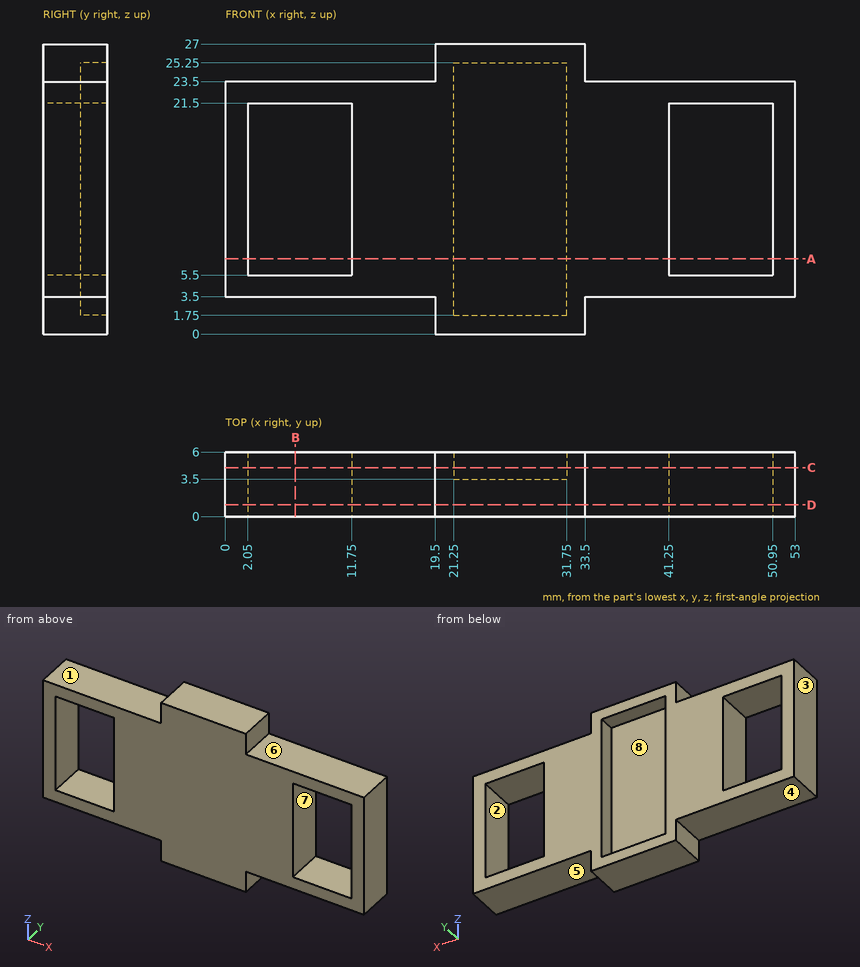
Study the drawing (mm; zero at the part's minimum x, y, z) and answer. A direction names the side the tool comes from. Round coordinates to 2 decimals unless told otherwise and drop trailing zeros. Write each loop counter-clockwise with the first axis right and the second up, starting at its lowest first coordinate (ties: lowest second). Pieces come first, ordered by that corner, then holes. Notation, with made-up numbers: (20, 47) - (65, 47) arc R13 ccw to (65, 64) - close; hole circle Ø9 at (-7.5, -20). An arc over 180 degrees is marked (long way). Return JSON: item names as keys, results as strings. Group by question number.
Q1. The part is cut by section D-D on y = 1.1. Write down the section's boundary in (x, z), then the cut area to 3 significant figures.
Q2. Each of these flat-tipped pins is pushed along its axis until it touches: pin 1 Ø3 at (x, y) = (11, 2.5) entering from +Z; pin 2 Ø1 at (x, y) = (42, 4) entering from -Z; pin 3 Ø1.5 at (x, z) = (24, 14) entering from +Y. Where does it stop, or does it pass through?
Q3. For the marked faces 4, 5, 6, 7 and 8, determine the directions among +Z, -Z, +X, -X, +Y, -Y from which every point of the face is accessible in a straight line to the end or side of a thin tool.
Q4. The part is cut by section B-B on x = 6.5. Write down the section's boundary in (y, z).
Q5. The mould has two halves that part along X. Classify the marked faces 1, 2 and 3: released by +X, released by -X, zero draft, split by the parting line, or undercut.
Q6. The part is cut by section A-A on z = 7. Write down the section's boundary in (x, y).
Q7. Find the intervals of material crossed by L1, parallel to X at y = 2.05, z = 8; L2, parallel to X at y = 5.5, z = 8.75; L3, parallel to Z at x = 29, y = 5.65, in increasing order.
Q8. The part is cut by section C-C on y = 4.55. Write down the section's boundary in (x, z).
Solved:
{
 "1": {"outline": "(0, 3.5) - (19.5, 3.5) - (19.5, 0) - (33.5, 0) - (33.5, 3.5) - (53, 3.5) - (53, 23.5) - (33.5, 23.5) - (33.5, 27) - (19.5, 27) - (19.5, 23.5) - (0, 23.5) - close; hole (2.05, 5.5) - (11.75, 5.5) - (11.75, 21.5) - (2.05, 21.5) - close; hole (41.25, 5.5) - (50.95, 5.5) - (50.95, 21.5) - (41.25, 21.5) - close", "area": "848 mm²"},
 "2": {"pin 1": "z = 23.5", "pin 2": "z = 3.5", "pin 3": "y = 3.5"},
 "3": {"face 4": "-Z, -X, +Y, -Y", "face 5": "-Z, +X, +Y, -Y", "face 6": "+Z, +X, +Y, -Y", "face 7": "+Y, -Y", "face 8": "+Y"},
 "4": {"outline": "(0, 3.5) - (6, 3.5) - (6, 5.5) - (0, 5.5) - close; (0, 21.5) - (6, 21.5) - (6, 23.5) - (0, 23.5) - close"},
 "5": {"face 1": "zero draft", "face 2": "undercut", "face 3": "released by -X"},
 "6": {"outline": "(0, 0) - (2.05, 0) - (2.05, 6) - (0, 6) - close; (11.75, 0) - (41.25, 0) - (41.25, 6) - (31.75, 6) - (31.75, 3.5) - (21.25, 3.5) - (21.25, 6) - (11.75, 6) - close; (50.95, 0) - (53, 0) - (53, 6) - (50.95, 6) - close"},
 "7": {"L1": "0 to 2.05, 11.75 to 41.25, 50.95 to 53", "L2": "0 to 2.05, 11.75 to 21.25, 31.75 to 41.25, 50.95 to 53", "L3": "0 to 1.75, 25.25 to 27"},
 "8": {"outline": "(0, 3.5) - (19.5, 3.5) - (19.5, 0) - (33.5, 0) - (33.5, 3.5) - (53, 3.5) - (53, 23.5) - (33.5, 23.5) - (33.5, 27) - (19.5, 27) - (19.5, 23.5) - (0, 23.5) - close; hole (2.05, 5.5) - (11.75, 5.5) - (11.75, 21.5) - (2.05, 21.5) - close; hole (21.25, 1.75) - (31.75, 1.75) - (31.75, 25.25) - (21.25, 25.25) - close; hole (41.25, 5.5) - (50.95, 5.5) - (50.95, 21.5) - (41.25, 21.5) - close"}
}
